Read the model definition and answer for the solid it produces. Units are mm, in the model's axes. Face numbers are marked on the shaded views. A direction names the side the tool comes from. Coordinates: 2 decimals unless noted, no trailing zeros. Order: outer loops, then holes, each group sorted by start corner. A loop starts at its lowest first (then second) coordinate and runs counter-clockwise, first axis right, second up. Notation, with made-up numbers: (28.25, -18) -> (60.25, -18) arc R25 ccw to (60.25, -3) -> close; hole circle Ø2 at (50.25, 27.5). An arc over 180 degrees is marked (long way). Answer as a JSON object with one key per item and string values. Group by question number.
1) Section C-C on x = 0 is taken. Determine the outline of the cut face in (y, z) (3 decimals), and give its area (3 significant figures).
2) Section B-B on y = 14.75 is taken. Determine the outline of the cut face in (x, z) (3 decimals).
3) A tool of negligible diameter and unlimited length cuts with its end or side. For the marked faces 5, 6 and 7, from which of +Z, -Z, +X, -X, +Y, -Y can it reach the whole face along a straight path? Write none if from no direction.
4) Section A-A on z = 4.5 is taken. Determine the outline of the cut face in (x, y) (3 decimals), and give its area (3 significant figures).
5) Determine the mould class of the marked faces 1, 2, 3 and 4 for opening direction X: released by +X, released by -X, zero draft, split by the parting line, or undercut.
6) Consider L1, parallel to X at y = 6.5, z = 7; L2, parallel to X at y = 13, z = 28.5 (3 decimals); L3, parallel to X at y = 7.75, z = 2.5. Determine where each line is inside the solid, lowest interval first.
7) Section D-D on x = 20 is taken. Determine the outline of the cut face in (y, z), and give its area (3 significant figures).
8) Given pin 1 (3 mm diameter, centred on x = 13, y = 4, fed in from +Z); pin 2 (6 mm diameter, centred on y = 6, z = 11.5, fed in from +X); pin 3 (6 mm diameter, centred on y = 9.5, z = 16.5, fed in from +X); pin 4 (3 mm diameter, centred on x = -20.98, y = 8.02, fed in from -Z), each flat-ended and moving along its own axis, determine where each tip first touches the part or whether it passes through.
from build123d import *

# Parameters (mm, degrees)
SKETCH_1_R             = 17.63
SKETCH_1_R_2           = 14.34
EXTRUDE_1_DEPTH        = 16.05
EXTRUDE_1_2_DEPTH      = 9.77
EXTRUDE_1_2_DEPTH_BACK = 3
SKETCH_2_W             = 16
SKETCH_2_H             = 16.05
SKETCH_3_W             = 3.41
SKETCH_3_H             = 16
CUT_EXTRUDE_1_DEPTH    = 37.411121927
SKETCH_4_R             = 1.91
CUT_EXTRUDE_2_DEPTH    = 39.675463798
EXTRUDE_2_DEPTH        = 4
EXTRUDE_2_DEPTH_BACK   = 2.77
SKETCH_5_W             = 12.19
SKETCH_5_H             = 8.263625949
SKETCH_6_W             = 12.19
SKETCH_6_H             = 6.77
EXTRUDE_3_DEPTH        = 63
SKETCH_8_W             = 12.19
SKETCH_8_H             = 6.77
EXTRUDE_4_DEPTH        = 0.16
EXTRUDE_5_DEPTH        = 3.16
EXTRUDE_5_DEPTH_BACK   = 10
SKETCH_12_W            = 16
SKETCH_12_H            = 16.05
SKETCH_13_W            = 1.21
SKETCH_13_H            = 16
CUT_EXTRUDE_3_DEPTH    = 73.543164889
SKETCH_14_R            = 1.91
CUT_EXTRUDE_4_DEPTH    = 90.07387176
SKETCH_15_R            = 4.05
CUT_EXTRUDE_5_DEPTH    = 24
SKETCH_16_W            = 56.400519221
SKETCH_16_H            = 19.935010357
CUT_EXTRUDE_6_DEPTH    = 73.088971918
SKETCH_17_W            = 12.19
SKETCH_17_H            = 71.423625949
EXTRUDE_7_DEPTH        = 25
SKETCH_18_W            = 26.793372528
SKETCH_18_H            = 63.398625949
CUT_EXTRUDE_7_DEPTH    = 25
SKETCH_19_R            = 4
CUT_EXTRUDE_8_DEPTH    = 24
CUT_EXTRUDE_9_DEPTH    = 29
SKETCH_21_W            = 8
SKETCH_21_H            = 16
CUT_EXTRUDE_10_DEPTH   = 8
EXTRUDE_9_DEPTH        = 2
FILLET_1_R             = 10


with BuildPart() as part:
    # 草圖1 → Extrude 1 (new body)
    with BuildSketch(Plane(origin=(0, 0, 0), x_dir=(1, 0, 0), z_dir=(0, 1, 0))):
        Circle(SKETCH_1_R)
        Circle(SKETCH_1_R_2, mode=Mode.SUBTRACT)
    extrude(amount=EXTRUDE_1_DEPTH)

    # 草圖2 → Extrude 1 2 (add, two sides: drawn at the far end of the back side and taken through both)
    with BuildSketch(Plane(origin=(17.75, 0, 0), x_dir=(0, 0, -1), z_dir=(1, 0, 0)).offset(-EXTRUDE_1_2_DEPTH_BACK)):
        with Locations((0, 8.025)):
            Rectangle(SKETCH_2_W, SKETCH_2_H)
    extrude(amount=EXTRUDE_1_2_DEPTH + EXTRUDE_1_2_DEPTH_BACK)

    # 草圖3 → 除料-伸長1 (cut, through all)
    with BuildSketch(Plane(origin=(0, 16.05, 0), x_dir=(1, 0, 0), z_dir=(0, 1, 0))):
        with Locations((25.815, 0)):
            Rectangle(SKETCH_3_W, SKETCH_3_H)
    extrude(amount=-CUT_EXTRUDE_1_DEPTH, mode=Mode.SUBTRACT)

    # 草圖4 → 除料-伸長2 (cut, through all)
    with BuildSketch(Plane.XY.offset(8)):
        with Locations((19.910203689, 8.025)):
            Circle(SKETCH_4_R)
    extrude(amount=-CUT_EXTRUDE_2_DEPTH, mode=Mode.SUBTRACT)

    # 草圖5 → 填料-伸長2 (add, two sides: drawn at the far end of the back side and taken through both)
    with BuildSketch(Plane.XY.offset(17.75).offset(-EXTRUDE_2_DEPTH_BACK)):
        with Locations((0, 12.156812974)):
            Rectangle(SKETCH_5_W, SKETCH_5_H)
    extrude(amount=EXTRUDE_2_DEPTH + EXTRUDE_2_DEPTH_BACK)

    # 草圖6 → 填料-伸長3 (add)
    with BuildSketch(Plane(origin=(0, 16.288625949, 0), x_dir=(1, 0, 0), z_dir=(0, 1, 0))):
        with Locations((0, -18.365)):
            Rectangle(SKETCH_6_W, SKETCH_6_H)
    extrude(amount=EXTRUDE_3_DEPTH)

    # 草圖8 → 填料-伸長4 (add)
    with BuildSketch(Plane(origin=(0, 79.288625949, 0), x_dir=(1, 0, 0), z_dir=(0, 1, 0))):
        with Locations((0, -18.365)):
            Rectangle(SKETCH_8_W, SKETCH_8_H)
    extrude(amount=EXTRUDE_4_DEPTH)

    # 草圖12 → 填料-伸長5 (add, two sides: drawn at the far end of the back side and taken through both)
    with BuildSketch(Plane(origin=(-17.75, 0, 0), x_dir=(0, 0, -1), z_dir=(1, 0, 0)).offset(-EXTRUDE_5_DEPTH_BACK)):
        with Locations((0.543544944, 8.025)):
            Rectangle(SKETCH_12_W, SKETCH_12_H)
    extrude(amount=EXTRUDE_5_DEPTH + EXTRUDE_5_DEPTH_BACK)

    # 草圖13 → 除料-伸長3 (cut, through all)
    with BuildSketch(Plane(origin=(0, 16.05, 0), x_dir=(1, 0, 0), z_dir=(0, 1, 0))):
        with Locations((-27.145, 0.543544944)):
            Rectangle(SKETCH_13_W, SKETCH_13_H)
    extrude(amount=-CUT_EXTRUDE_3_DEPTH, mode=Mode.SUBTRACT)

    # 草圖14 → 除料-伸長4 (cut, through all)
    with BuildSketch(Plane(origin=(0, 0, -8.543544944), x_dir=(-1, 0, 0), z_dir=(0, 0, -1))):
        with Locations(Location((20.980783679, 8.025, 0), (0, 0, 90))):
            Circle(SKETCH_14_R)
    extrude(amount=-CUT_EXTRUDE_4_DEPTH, mode=Mode.SUBTRACT)

    # 草圖15 → 除料-伸長5 (cut)
    with BuildSketch(Plane(origin=(0, 79.448625949, 0), x_dir=(1, 0, 0), z_dir=(0, 1, 0))):
        with Locations((0, -14.98)):
            Circle(SKETCH_15_R)
    extrude(amount=-CUT_EXTRUDE_5_DEPTH, mode=Mode.SUBTRACT)

    # 草圖16 → 除料-伸長6 (cut, through all)
    with BuildSketch(Plane(origin=(0, 16.05, 0), x_dir=(1, 0, 0), z_dir=(0, 1, 0))):
        with Locations((-4.090259611, 9.967505179)):
            Rectangle(SKETCH_16_W, SKETCH_16_H)
    extrude(amount=-CUT_EXTRUDE_6_DEPTH, mode=Mode.SUBTRACT)

    # 草圖17 → 填料-伸長7 (add)
    with BuildSketch(Plane.XY.offset(21.75)):
        with Locations((0, 43.736812975)):
            Rectangle(SKETCH_17_W, SKETCH_17_H)
    extrude(amount=EXTRUDE_7_DEPTH)

    # 草圖18 → 除料-伸長7 (cut)
    with BuildSketch(Plane.ZY.offset(6.095)):
        with Locations((28.376686264, 47.749312975)):
            Rectangle(SKETCH_18_W, SKETCH_18_H)
    extrude(amount=-CUT_EXTRUDE_7_DEPTH, mode=Mode.SUBTRACT)

    # 草圖19 → 除料-伸長8 (cut)
    with BuildSketch(Plane(origin=(0, 79.448625949, 0), x_dir=(1, 0, 0), z_dir=(0, 1, 0))):
        with Locations((0, -41.773372528)):
            Circle(SKETCH_19_R)
    extrude(amount=-CUT_EXTRUDE_8_DEPTH, mode=Mode.SUBTRACT)

    # 草圖20 → 除料-伸長9 (cut)
    with BuildSketch(Plane(origin=(6.095, 0, 0), x_dir=(0, 0, -1), z_dir=(1, 0, 0))):
        Polygon((-41.773372528, 16.05), (-41.773372528, 8.025), (-46.75, 8.025), (-46.75, 79.448625949), (-41.773372528, 79.448625949), align=None)
    extrude(amount=-CUT_EXTRUDE_9_DEPTH, mode=Mode.SUBTRACT)

    # 草圖21 → 除料-伸長10 (cut)
    with BuildSketch(Plane(origin=(0, 16.05, 0), x_dir=(1, 0, 0), z_dir=(0, 1, 0))):
        with Locations((0, -28)):
            Rectangle(SKETCH_21_W, SKETCH_21_H)
    extrude(amount=-CUT_EXTRUDE_10_DEPTH, mode=Mode.SUBTRACT)

    # 草圖23 → 填料-伸長9 (add)
    with BuildSketch(Plane.XZ.offset(-8.025)):
        Polygon((-6.095, 41.773372528), (-6.095, 17.75), (6.13829314, 17.75), (6.095, 41.773372528), align=None)
    extrude(amount=EXTRUDE_9_DEPTH)

    # 圓角1
    # the kernel refuses this fillet: 10 mm, written as the material it takes off along each edge
    with BuildSketch(Plane(origin=(-21.095, 6.025, 17.75), x_dir=(0, 0, 1), z_dir=(1, 0, 0))) as fillet_1_piece_1:
        with BuildLine():
            CenterArc((6, -10), FILLET_1_R, 90, 36.869897646)
            Line((0, -2), (0, 0))
            Line((0, 0), (6, 0))
        make_face()
    extrude(amount=42.23329314, mode=Mode.SUBTRACT)


solid = part.part
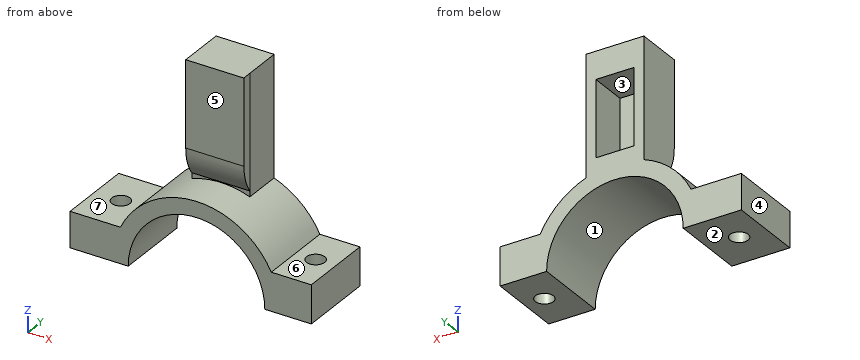
Worked answers:
{
 "1": {"outline": "(0, 14.34) -> (16.05, 14.34) -> (16.05, 20) -> (8.05, 20) -> (8.05, 36) -> (16.05, 36) -> (16.05, 41.773) -> (6.025, 41.773) -> (6.025, 23.75) arc R10 ccw to (8.025, 17.75) -> (8.025, 17.63) -> (0, 17.63) -> close", "area": "163 mm²"},
 "2": {"outline": "(-26.54, 0) -> (-14.34, 0) arc R14.34 cw to (14.34, 0) -> (24.11, 0) -> (24.11, 8) -> (15.71, 8) arc R17.63 ccw to (6.095, 16.543) -> (6.095, 41.773) -> (-6.095, 41.773) -> (-6.095, 16.543) arc R17.63 ccw to (-15.976, 7.456) -> (-26.54, 7.456) -> close; hole (-4, 20) -> (4, 20) -> (4, 36) -> (-4, 36) -> close"},
 "3": {"face 5": "+Z, +X, -X, -Y", "face 6": "+Z, +X, +Y, -Y", "face 7": "+Z, -X, +Y, -Y"},
 "4": {"outline": "(-26.54, 0) -> (-13.616, 0) -> (-13.616, 16.05) -> (-26.54, 16.05) -> close; (13.616, 0) -> (24.11, 0) -> (24.11, 16.05) -> (13.616, 16.05) -> close; hole circle Ø3.82 at (-20.981, 8.025); hole circle Ø3.82 at (19.91, 8.025)", "area": "353 mm²"},
 "5": {"face 1": "undercut", "face 2": "zero draft", "face 3": "undercut", "face 4": "released by -X"},
 "6": {"L1": "x = -26.54 to -22.13, -19.83 to -12.52, 12.52 to 18.76, 21.06 to 24.11", "L2": "x = -6.095 to -4, 4 to 6.095", "L3": "x = -26.54 to -22.87, -19.09 to -14.12, 14.12 to 18.02, 21.8 to 24.11"},
 "7": {"outline": "(0, 0) -> (6.12, 0) -> (6.12, 8) -> (0, 8) -> close; (9.93, 0) -> (16.05, 0) -> (16.05, 8) -> (9.93, 8) -> close", "area": "97.9 mm²"},
 "8": {"pin 1": "stops at z = 13.36", "pin 2": "stops at x = 15.45", "pin 3": "stops at x = 11.34", "pin 4": "passes through"}
}
